Read the model definition and answer for the solid it produces. Units are mm, in the model's axes. Round coordinates to 2 decimals unless told otherwise and drop trailing zeros. Order: outer loops, then holes, each group sorted by start corner. A loop starts at its lowest first (then second) coordinate and runs counter-clockwise, first axis right, second up. Notation, with made-up numbers: (-32.5, -32) - (8.5, -32) arc R21 ccw to (8.5, 5) - close; hole circle Ø1 at (52.5, 24). An arc over 180 degrees is marked (long way). Answer as a JSON object with one key per item and string values. Group by question number.
Q1. Given pin 1 Ø1.5 at (y, z) = (-57, 1.5) entering from +X; pin 2 Ø1.4 at (x, z) = (22.5, 1.5) entering from -Y; pin 3 Ø1.5 at (y, z) = (-58.5, 1.5) entering from -X, each flat-ended and moving along its own axis, determine where each tip first touches the part or whether it passes through.
Q2. A cutting plane is placed at B-B on y = 21. Determine the outline of the cut face in (x, z), and give its area (3 significant figures).
Q3. A cutting plane is placed at D-D on x = 62. Determine the outline of the cut face in (y, z).
Q4. A cutting plane is placed at C-C on x = -2. Determine the outline of the cut face in (y, z).
Q5. Consider line 1 (Y direction, x = 0, z = 2.15); line 2 (Y direction, x = -31.5, z = 0.35); line 3 (X direction, y = 58, z = 1.75). Determine where each line is inside the solid, lowest interval first.
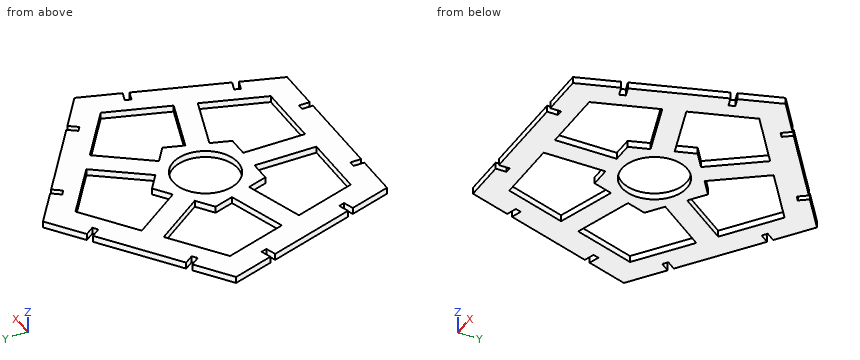
```python
from build123d import *

# Parameters (mm, degrees)
F1_DEPTH = 3
F2_R     = 15
F3_DEPTH = 3


with BuildPart() as f1:
    # F0 (on Top) → F1 (new body)
    with BuildSketch(Plane.XY):
        Polygon((16.18034, 63.244295), (0, 75), (-16.18034, 63.244295), (-13.241414, 59.19921), (-15.506661, 57.553411), (-18.445587, 61.598496), (-52.883651, 36.577778), (-49.944725, 32.532693), (-52.209973, 30.886895), (-55.148899, 34.93198), (-71.329239, 23.176275), (-65.148899, 4.155144), (-60.393616, 5.700229), (-59.528369, 3.037271), (-64.283651, 1.492186), (-51.129481, -38.992186), (-46.374199, -37.447101), (-45.508951, -40.110059), (-50.264234, -41.655144), (-44.083894, -60.676275), (-24.083894, -60.676275), (-24.083894, -55.676275), (-21.283894, -55.676275), (-21.283894, -60.676275), (21.283894, -60.676275), (21.283894, -55.676275), (24.083894, -55.676275), (24.083894, -60.676275), (44.083894, -60.676275), (50.264234, -41.655144), (45.508951, -40.110059), (46.374199, -37.447101), (51.129481, -38.992186), (64.283651, 1.492186), (59.528369, 3.037271), (60.393616, 5.700229), (65.148899, 4.155144), (71.329239, 23.176275), (55.148899, 34.93198), (52.209973, 30.886895), (49.944725, 32.532693), (52.883651, 36.577778), (18.445587, 61.598496), (15.506661, 57.553411), (13.241414, 59.19921), align=None)
        Polygon((-57.063391, 18.54102), (0, 60), (57.063391, 18.54102), (35.267115, -48.54102), (-35.267115, -48.54102), align=None, mode=Mode.SUBTRACT)
    extrude(amount=F1_DEPTH)

    # F2 (on face) → F3 (join)
    with BuildSketch(Plane.XY.offset(3)):
        Polygon((5, -20), (14.530851, -20), (17.476045, -10.935622), (44.620168, -19.755283), (47.710338, -10.244717), (20.566215, -1.425057), (23.51141, 7.63932), (15.80079, 13.241414), (32.57678, 36.331584), (24.486611, 42.209436), (7.71062, 19.119266), (0, 24.72136), (-7.71062, 19.119266), (-24.486611, 42.209436), (-32.57678, 36.331584), (-15.80079, 13.241414), (-23.51141, 7.63932), (-20.566215, -1.425057), (-47.710338, -10.244717), (-44.620168, -19.755283), (-17.476045, -10.935622), (-14.530851, -20), (-5, -20), (-5, -48.54102), (5, -48.54102), align=None)
        Circle(F2_R, mode=Mode.SUBTRACT)
    extrude(amount=-F3_DEPTH)


solid = f1.part
```
Result set:
{
 "1": {"pin 1": "stops at x = 45.52", "pin 2": "stops at y = -55.68", "pin 3": "stops at x = -45.03"},
 "2": {"outline": "(-70.62, 0) - (-53.68, 0) - (-53.68, 3) - (-70.62, 3) - close; (-21.44, 0) - (-9.08, 0) - (-9.08, 3) - (-21.44, 3) - close; (-5.12, 0) - (5.12, 0) - (5.12, 3) - (-5.12, 3) - close; (9.08, 0) - (21.44, 0) - (21.44, 3) - (9.08, 3) - close; (53.68, 0) - (70.62, 0) - (70.62, 3) - (53.68, 3) - close", "area": "207 mm²"},
 "3": {"outline": "(-5.54, 0) - (2.23, 0) - (2.23, 3) - (-5.54, 3) - close; (5.18, 0) - (29.95, 0) - (29.95, 3) - (5.18, 3) - close"},
 "4": {"outline": "(-60.68, 0) - (-14.87, 0) - (-14.87, 3) - (-60.68, 3) - close; (14.87, 0) - (23.27, 0) - (23.27, 3) - (14.87, 3) - close; (58.55, 0) - (73.55, 0) - (73.55, 3) - (58.55, 3) - close"},
 "5": {"line 1": "y = -60.68 to -15, 15 to 24.72, 60 to 75", "line 2": "y = -60.68 to -48.54, -15.49 to -4.98, 34.85 to 52.11", "line 3": "x = -23.4 to -15.83, -14.89 to -2.75, 2.75 to 14.89, 15.83 to 23.4"}
}
